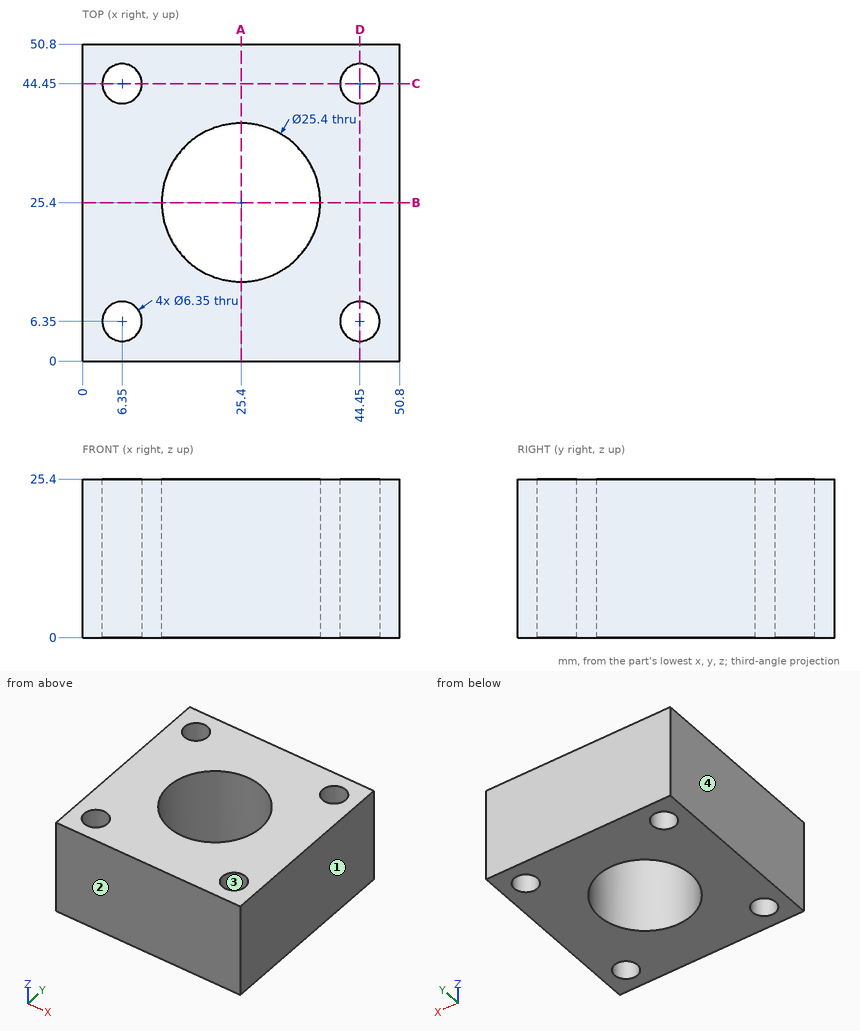
The figure shows three views and two pictorial views of one solid part (mm, origin at its lowest corner). Answer the questions. Give positions to 0.01 mm unless a question says otherwise; leave off trailing zeros. Write each loop counter-clockwise with the first axis right and the second up, starting at its lowest first coordinate (ties: lowest second). Pieces come first, ordered by that corner, then holes. Notation, with made-up numbers: (21, 26.5) - (47, 26.5) arc R13 ccw to (47, 39.5) - close; hole circle Ø3 at (-16.75, 56.25). An arc over 180 degrees is marked (long way). Return JSON: item names as keys, results as strings.
Q1. Given P1, Ø4, axis at x = 6.35, y = 44.45, coming from the +Z side, flat-ended and moving along its own axis, determine where the tip first touches the part or whether it passes through.
Reply:
{"P1": "through"}
Q2. Consider line 1 along Y through (x, z) = (6.35, 17.75) (3 decimals); line 2 along X through (y, z) = (42, 14.5); line 3 along Y through (x, z) = (15.5, 18.25). Determine where each line is inside the solid, lowest interval first. Write a range as [from, to].
Reply:
{"line 1": "[0, 3.175], [9.525, 41.275], [47.625, 50.8]", "line 2": "[0, 4.33], [8.37, 42.43], [46.47, 50.8]", "line 3": "[0, 17.45], [33.35, 50.8]"}
Q3. For a pull along X with two mould halves and no side action, classify the marked faces 1, 2, 3 and 4 as released by +X, released by -X, zero draft, split by the parting line, or undercut.
Reply:
{"face 1": "released by +X", "face 2": "zero draft", "face 3": "undercut", "face 4": "released by -X"}
Q4. A cutting plane is placed at C-C, the plane y = 44.45. Determine the outline of the cut face in (x, z) (3 decimals).
Reply:
{"outline": "(0, 0) - (3.175, 0) - (3.175, 25.4) - (0, 25.4) - close; (9.525, 0) - (41.275, 0) - (41.275, 25.4) - (9.525, 25.4) - close; (47.625, 0) - (50.8, 0) - (50.8, 25.4) - (47.625, 25.4) - close"}
Q5. A cutting plane is placed at A-A, the plane x = 25.4. Determine the outline of the cut face in (y, z), and give its area (3 significant figures).
Reply:
{"outline": "(0, 0) - (12.7, 0) - (12.7, 25.4) - (0, 25.4) - close; (38.1, 0) - (50.8, 0) - (50.8, 25.4) - (38.1, 25.4) - close", "area": "645 mm²"}
